from build123d import *

# Parameters (mm, degrees)
PAD101_DEPTH    = 2
PAD102_DEPTH    = 6.75
SKETCH142_W     = 2
SKETCH142_H     = 23
SKETCH142_W_2   = 21
SKETCH142_H_2   = 2
POCKET042_DEPTH = 1
SKETCH143_W     = 10
SKETCH143_H     = 10
PAD103_DEPTH    = 5
SKETCH144_R     = 2.5
POCKET043_DEPTH = 5
SKETCH145_W     = 20
SKETCH145_H     = 20
PAD104_DEPTH    = 5
SKETCH146_R     = 2.7
POCKET044_DEPTH = 8.751
PAD105_DEPTH    = 23
PAD106_DEPTH    = 3.75
POCKET045_DEPTH = 5.001
PAD107_DEPTH    = 20
SKETCH148_W     = 20
SKETCH148_H     = 5
PAD108_DEPTH    = 20
PAD109_DEPTH    = 14
SKETCH149_R     = 2.7
POCKET046_DEPTH = 5
FILLET021_R     = 5
FILLET022_R     = 2.99
FILLET023_R     = 1
PAD110_DEPTH    = 12


with BuildPart() as body050:
    # Sketch140 → Pad101 (new body)
    with BuildSketch(Plane.XY):
        Polygon((-23, 18), (-23, 0), (0, 0), (0, 13), (23, 13), (23, 26), (-7, 26), (-9, 26), (-9, 21), (-13, 20), (-23, 20), align=None)
    extrude(amount=PAD101_DEPTH)

    # Sketch141 (on Face13 of Pad101) → Pad102 (join)
    with BuildSketch(Plane.XY.offset(2)):
        Polygon((-23, 0), (0, 0), (0, 13), (23, 13), (23, 26), (-9, 26), (-9, 21), (-13, 20), (-23, 20), (-23, 18), (-13, 18), (-7, 19), (-7, 25), (21, 25), (21, 15), (-2, 15), (-2, 2), (-23, 2), align=None)
    extrude(amount=PAD102_DEPTH)

    # Sketch142 (on Face7 of Pad102) → Pocket042 (cut)
    with BuildSketch(Plane.XY.offset(2)):
        with Locations((-6, 13.5)):
            Rectangle(SKETCH142_W, SKETCH142_H)
        with Locations((6.5, 17)):
            Rectangle(SKETCH142_W_2, SKETCH142_H_2)
    extrude(amount=-POCKET042_DEPTH, mode=Mode.SUBTRACT)

    # Sketch143 (on Face18 of Pocket042) → Pad103 (join)
    with BuildSketch(Plane.XY.offset(8.75)):
        with Locations((5, 8)):
            Rectangle(SKETCH143_W, SKETCH143_H)
    extrude(amount=-PAD103_DEPTH)

    # Sketch144 (on Face29 of Pad103) → Pocket043 (cut)
    with BuildSketch(Plane.XY.offset(8.75)):
        with Locations((5, 8)):
            Circle(SKETCH144_R)
    extrude(amount=-POCKET043_DEPTH, mode=Mode.SUBTRACT)

    # Sketch145 (on Face4 of Pocket043) → Pad104 (join)
    with BuildSketch(Plane(origin=(0, 0, 0), x_dir=(1, 0, 0), z_dir=(0, 0, -1))):
        with Locations((33, -16)):
            Rectangle(SKETCH145_W, SKETCH145_H)
    extrude(amount=-PAD104_DEPTH)

    # Sketch146 (on Face13 of Pad104) → Pocket044 (cut, through all)
    with BuildSketch(Plane(origin=(0, 0, 0), x_dir=(1, 0, 0), z_dir=(0, 0, -1))):
        with Locations((33, -16)):
            Circle(SKETCH146_R)
    extrude(amount=-POCKET044_DEPTH, mode=Mode.SUBTRACT)

    # Pocket044 Face25 → Pad105 (add)
    with BuildSketch(Plane(origin=(23, 9.5, 2.5), x_dir=(0, 1, 0), z_dir=(-1, 0, 0))):
        Polygon((3.5, 2.5), (-3.5, 2.5), (-3.5, -2.5), (3.5, -2.5), (3.5, 0.5), align=None)
    extrude(amount=PAD105_DEPTH)

    # Pad105 Face46 → Pad106 (add)
    with BuildSketch(Plane(origin=(5, 4.454221, 3.75), x_dir=(0, -1, 0), z_dir=(0, 0, -1))):
        with BuildLine():
            Line((-1.545779, 5), (-1.545779, 1.5))
            ThreePointArc((-1.545779, 1.5), (-1.045779, 0), (-1.545779, -1.5))
            Line((-1.545779, -1.5), (-1.545779, -5))
            Line((-1.545779, -5), (1.454221, -5))
            Line((1.454221, -5), (1.454221, 5))
            Line((1.454221, 5), (-1.545779, 5))
        make_face()
    extrude(amount=PAD106_DEPTH)

    # Pad106 Face53 → Pocket045 (cut, through all)
    with BuildSketch(Plane(origin=(5, 8.120883, 5), x_dir=(0, 1, 0), z_dir=(0, 0, 1))):
        with BuildLine():
            ThreePointArc((-2.120883, -1.5), (-1.238917, -2.236068), (-0.120883, -2.5))
            ThreePointArc((-0.120883, -2.5), (2.115185, 1.118034), (-2.120883, 1.5))
            Line((-2.120883, 1.5), (-2.120883, -1.5))
        make_face()
    extrude(amount=-POCKET045_DEPTH, mode=Mode.SUBTRACT)

    # Sketch147 (on Face1 of Pocket045) → Pad107 (join)
    with BuildSketch(Plane(origin=(-23, 0, 0), x_dir=(0, -1, 0), z_dir=(-1, 0, 0))):
        Polygon((-26, 0), (-26, 5), (-18, 5), (-18, 2), (-6, 2), (-6, 0), align=None)
    extrude(amount=PAD107_DEPTH)

    # Sketch148 (on Face24 of Pad107) → Pad108 (join)
    with BuildSketch(Plane(origin=(-43, 0, 0), x_dir=(0, -1, 0), z_dir=(-1, 0, 0))):
        with Locations((-16, 2.5)):
            Rectangle(SKETCH148_W, SKETCH148_H)
    extrude(amount=PAD108_DEPTH)

    # Pad108 Face26 → Pad109 (add)
    with BuildSketch(Plane(origin=(-23, 23, 2.5), x_dir=(0, -1, 0), z_dir=(1, 0, 0))):
        Polygon((3, -2.5), (3, 0.5), (3, 2.5), (-3, 2.5), (-3, -2.5), align=None)
    extrude(amount=PAD109_DEPTH)

    # Sketch149 (on Face57 of Pad109) → Pocket046 (cut)
    with BuildSketch(Plane.XY.offset(5)):
        with Locations((-53, 16)):
            Circle(SKETCH149_R)
    extrude(amount=-POCKET046_DEPTH, mode=Mode.SUBTRACT)

    # Fillet021
    fillet021_edges = [body050.edges().sort_by_distance(p)[0] for p in [
        (-63, 26, 2.5),
        (-63, 6, 2.5),
        (43, 26, 2.5),
        (43, 6, 2.5),
    ]]
    fillet(fillet021_edges, radius=FILLET021_R)

    # Fillet022
    fillet022_edges = [body050.edges().sort_by_distance(p)[0] for p in [
        (10, 3, 1.875),
        (10, 3, 6.25),
    ]]
    fillet(fillet022_edges, radius=FILLET022_R)

    # Fillet023
    fillet023_edges = [body050.edges().sort_by_distance(p)[0] for p in [
        (-23, 0, 1),
        (-23, 0, 5.375),
        (0, 0, 5.375),
        (0, 0, 1),
        (23, 13, 6.875),
        (23, 26, 6.875),
        (-9, 26, 6.875),
        (-23, 20, 6.875),
    ]]
    fillet(fillet023_edges, radius=FILLET023_R)

    # Sketch150 (on Face26 of Fillet023) → Pad110 (join)
    with BuildSketch(Plane.XZ.offset(-6)):
        Polygon((-43, 5), (-43, 2), (-38, 2), align=None)
    extrude(amount=-PAD110_DEPTH)


with BuildPart() as part_mirroring003:
    # Part__Mirroring003: instance of Body050
    add(body050.part.mirror(Plane(origin=(0, 13, 0), x_dir=(0, 1, 0), z_dir=(0, 0, 1))))


with BuildPart() as part_mirroring003_1:
    # Part__Mirroring003 placement: moved
    add(part_mirroring003.part.moved(Location((0, 0, 17.5))))


solid = part_mirroring003_1.part
For this review, take the finished solid that the model builds, in its own axes (mm). A direction names the side the tool comes from. Round coordinates to 2 decimals unless told otherwise and drop trailing zeros. Loops run counter-clockwise (first coordinate to the right, second up) from the corner with the lowest first, then second, coordinate; pieces in that order, holes last. Notation, with made-up numbers: (-40, 8.5) - (-7, 8.5) arc R27 ccw to (-7, 35.5) - close; hole circle Ø8 at (75.25, 38.25). An arc over 180 degrees is marked (long way). Use one line per item in the form item = value.
Item 1: Mouldability with a two-part tool opening along X and no side actions: class faces 1 (the cylindrical face through (-61, 25, 15)), 2 (the flat face through (-17, 20, 11)), 3 (the cylindrical face through (9.15, 3.9, 13.19)), 4 (the flat face through (-10, 18.5, 12.2)) as +X half, -X half, draft (parallel to the pull), parting line (faces both ways), or undercut.
Answers:
face_1 = -X half
face_2 = draft
face_3 = +X half
face_4 = undercut
Item 2: Consider section D-D on x = 34.5. Write out the cut boundary in (y, z) (3 decimals).
Answers:
outline = (6, 12.5) - (13.755, 12.5) - (13.755, 17.5) - (6, 17.5) - close; (18.245, 12.5) - (26, 12.5) - (26, 17.5) - (18.245, 17.5) - close
Item 3: Consider section A-A on z = 10.5. Write out the cut boundary in (x, y).
Answers:
outline = (-23, 1) arc R1 ccw to (-22, 0) - (-1, 0) arc R1 ccw to (0, 1) - (0, 3) - (7.01, 3) arc R2.99 ccw to (10, 5.99) - (10, 13) - (22, 13) arc R1 ccw to (23, 14) - (23, 25) arc R1 ccw to (22, 26) - (-8, 26) arc R1 ccw to (-9, 25) - (-9, 21) - (-13, 20) - (-22, 20) arc R1 ccw to (-23, 19) - (-23, 18) - (-13, 18) - (-7, 19) - (-7, 25) - (21, 25) - (21, 15) - (-2, 15) - (-2, 2) - (-23, 2) - close; hole circle Ø5 at (5, 8)
Item 4: Clearance check with flat-ended pins moving along their axes: P1, Ø6, axis at x = 33, y = 16, coming from the -Z side; P2, Ø3, axis at y = 15, z = 10, coming from the +X side; P3, Ø5, axis at x = 11.5, y = 7, coming from the -Z side; P4, Ø1.5, axis at y = 2.5, z = 15, coming from the -X side. State where each tip first meets the part, or that it passes through.
Answers:
P1 = 12.5
P2 = 23
P3 = 8.75
P4 = -23
Item 5: Consider section B-B on x = -53. Write out the cut boundary in (y, z).
Answers:
outline = (6, 12.5) - (13.3, 12.5) - (13.3, 17.5) - (6, 17.5) - close; (18.7, 12.5) - (26, 12.5) - (26, 17.5) - (18.7, 17.5) - close
Item 6: For line 1 (Y direction, x = 5, z = 12.5); line 2 (Y direction, x = -53, z = 13.8); line 3 (X direction, y = 6, z = 11.5), list the stretches that pass through material, from the lowest coordinate up.
Answers:
line_1 = 3 to 5.5, 10.5 to 15, 25 to 26
line_2 = 6 to 13.3, 18.7 to 26
line_3 = -2 to 3.5, 6.5 to 10
Item 7: Tool access review of faces 5 (the flat face through (21, 20, 12)), 6 (the flat face through (2, 11, 8.75)), 7 (the flat face through (-42, 18.4, 12.5)): name each direction out of +Z, -Z, +X, -X, +Y, -Y from which nothing blocks a thin tool from reaching the whole face with its end or side.
Answers:
face_5 = -Z
face_6 = -Z, +X, -X, +Y, -Y
face_7 = -Z, -X, +Y
